Geometry: final body of the model. Coordinates: model frame, mm. A direction names the side the tool comes from. Coordinates: 2 decimals unless noted, no trailing zeros. Loops run counter-clockwise (first coordinate to the right, second up) from the corner with the lowest first, then second, coordinate; pieces in that order, holes last. Notation, with made-up numbers: (61, 73.25) -> (100, 73.25) arc R14 ccw to (100, 82.25) -> close; hole circle Ø5 at (-40, 59.25). An arc over 180 degrees is marked (long way). One line per item, written item: value. Start each with the question number.
Item 1: Contact query for flat-ended pins moving along their axis: pin 1 Ø4 at (y, z) = (91, 13) entering from -X; pin 2 Ø20 at (x, z) = (-41, 20.5) entering from +Y; pin 3 Ø9 at (x, y) = (2.4, -141.6) entering from -Z; pin 4 Ø10 at (x, y) = (-69.5, 1) entering from +Z. Output: stop coordinate, or through.
Item 2: Ray query, probe 1 along X at (y, z) = (-3, 33.5); probe 2 along Y at (x, z) = (-1.5, 38); probe 3 along X at (y, z) = (-18, 20.5). Return the intervals inside material, ascending. Write a range as from..to.
Item 3: Section query C-C on x = 144. Return loops of the section in (y, z).
Item 4: Mould query, pull axis Y, two halves, no side actions, for faces 1 (the cylindrical face through (-144.186, -0.22, 2.465)), 2 (the flat face through (137, 0, 5)), 3 (the cylindrical face through (121.934, -50.557, 22.185)). Classes: +Y half, -Y half, draft (parallel to the pull), parting line (faces both ways), or undercut.
Item 5: Set-up query: faces 4 (the flat face through (-1, 84.992, 25)), 5 (the flat face through (5, 2, 0)). Return all of +Z, -Z, +X, -X, +Y, -Y with unobstructed straight access to the full face (end or side cutting, diameter ignored); none if empty.
Item 6: Section query A-A on y = 0. Return loops of the section in (x, z).
Item 7: Section query D-D on x = -19. Return loops of the section in (y, z).
Item 8: Section query B-B on z = 38.5. Return loops of the section in (x, y), then the cut area to 3 significant figures.
from build123d import *

# Parameters (mm, degrees)
SKETCH1_R           = 132
BOSS_EXTRUDE1_DEPTH = 5
SKETCH2_R           = 132
SKETCH2_R_2         = 128
BOSS_EXTRUDE2_DEPTH = 40
BOSS_EXTRUDE3_DEPTH = 40
SKETCH6_W           = 40
SKETCH6_H           = 20
BOSS_EXTRUDE5_DEPTH = 5
SKETCH7_W           = 40
SKETCH7_H           = 20
CUT_EXTRUDE1_DEPTH  = 5
SKETCH8_W           = 40
SKETCH8_H           = 10
BOSS_EXTRUDE7_DEPTH = 5
SKETCH9_R           = 5
BOSS_EXTRUDE8_DEPTH = 5
CIRPATTERN1_COUNT   = 4


with BuildPart() as part:
    # Sketch1 → Boss-Extrude1 (new body)
    with BuildSketch(Plane.XY):
        Circle(SKETCH1_R)
    extrude(amount=BOSS_EXTRUDE1_DEPTH)

    # Sketch2 → Boss-Extrude2 (add)
    with BuildSketch(Plane.XY.offset(5)):
        Circle(SKETCH2_R)
        Circle(SKETCH2_R_2, mode=Mode.SUBTRACT)
    extrude(amount=BOSS_EXTRUDE2_DEPTH)

    # Sketch3 → Boss-Extrude3 (add)
    with BuildSketch(Plane.XY.offset(5)):
        with BuildLine():
            ThreePointArc((95.710026061, 84.99171084), (0, 128), (-95.710026061, 84.99171084))
            Line((-95.710026061, 84.99171084), (95.710026061, 84.99171084))
        make_face()
        with BuildLine():
            Line((95.710026061, 84.99171084), (95.710026061, -84.99171084))
            ThreePointArc((95.710026061, -84.99171084), (119.655512484, -45.45941412), (128, 0))
            ThreePointArc((128, 0), (119.655512484, 45.45941412), (95.710026061, 84.99171084))
        make_face()
        with BuildLine():
            Line((95.710026061, -84.99171084), (-95.710026061, -84.99171084))
            ThreePointArc((-95.710026061, -84.99171084), (0, -128), (95.710026061, -84.99171084))
        make_face()
        with BuildLine():
            ThreePointArc((-95.710026061, 84.99171084), (-128, 0), (-95.710026061, -84.99171084))
            Line((-95.710026061, -84.99171084), (-95.710026061, 84.99171084))
        make_face()
    extrude(amount=BOSS_EXTRUDE3_DEPTH)

    # Sketch6 → Boss-Extrude5 (add)
    with BuildSketch(Plane.XY.offset(5)):
        with Locations((-50, 0)):
            Rectangle(SKETCH6_W, SKETCH6_H)
    extrude(amount=BOSS_EXTRUDE5_DEPTH)

    # Sketch7 → Cut-Extrude1 (cut)
    with BuildSketch(Plane.XY.offset(10)):
        with Locations((-50, 0)):
            Rectangle(SKETCH7_W, SKETCH7_H)
    extrude(amount=-CUT_EXTRUDE1_DEPTH, mode=Mode.SUBTRACT)

    # Sketch8 → Boss-Extrude7 (add)
    with BuildSketch(Plane.XY.offset(5)):
        with Locations((-75.710026061, -5)):
            Rectangle(SKETCH8_W, SKETCH8_H)
        with Locations((-75.710026061, 5)):
            Rectangle(SKETCH8_W, SKETCH8_H)
    extrude(amount=BOSS_EXTRUDE7_DEPTH)

    # Sketch9 → Boss-Extrude8 (add)
    with BuildSketch(Plane(origin=(0, 0, 0), x_dir=(-1, 0, 0), z_dir=(0, 0, -1))):
        with BuildLine():
            ThreePointArc((-129.632575758, -24.887653615), (-132, 0), (-129.632575758, 24.887653615))
            ThreePointArc((-129.632575758, 24.887653615), (-157, 0), (-129.632575758, -24.887653615))
        make_face()
        with Locations((-144, 0)):
            Circle(SKETCH9_R, mode=Mode.SUBTRACT)
    boss_extrude8 = extrude(amount=-BOSS_EXTRUDE8_DEPTH)

    # CirPattern1: Boss-Extrude8 ×4 about axis
    cirpattern1_axis = Axis((2.404422144, 0, 0), (0, 0, 1))
    for i in range(1, CIRPATTERN1_COUNT):
        add(boss_extrude8.rotate(cirpattern1_axis, i * 360 / CIRPATTERN1_COUNT))


solid = part.part
Reply:
1. pin 1: stops at x = -97.48
1. pin 2: stops at y = 128.31
1. pin 3: passes through
1. pin 4: stops at z = 10
2. probe 1: x = -131.97..-95.71, 95.71..131.97
2. probe 2: y = -131.99..-84.99, 84.99..131.99
2. probe 3: x = -130.77..-95.71, 95.71..130.77
3. outline: (-21.93, 0) -> (-5, 0) -> (-5, 5) -> (-21.93, 5) -> close; (5, 0) -> (21.93, 0) -> (21.93, 5) -> (5, 5) -> close
4. face 1: undercut
4. face 2: draft
4. face 3: parting line
5. face 4: +Z
5. face 5: -Z, +X, -X, +Y, -Y
6. outline: (-152.19, 0) -> (-144.19, 0) -> (-144.19, 5) -> (-152.19, 5) -> close; (-134.19, 0) -> (139, 0) -> (139, 5) -> (132, 5) -> (132, 45) -> (95.71, 45) -> (95.71, 5) -> (-55.71, 5) -> (-55.71, 10) -> (-95.71, 10) -> (-95.71, 45) -> (-132, 45) -> (-132, 5) -> (-134.19, 5) -> close; (149, 0) -> (157, 0) -> (157, 5) -> (149, 5) -> close
7. outline: (-142.51, 0) -> (142.51, 0) -> (142.51, 5) -> (130.63, 5) -> (130.63, 45) -> (84.99, 45) -> (84.99, 5) -> (-84.99, 5) -> (-84.99, 45) -> (-130.63, 45) -> (-130.63, 5) -> (-142.51, 5) -> close
8. outline: circle Ø264 at (0, 0); hole (-95.71, -84.99) -> (95.71, -84.99) -> (95.71, 84.99) -> (-95.71, 84.99) -> close
8. area: 22,200 mm²
